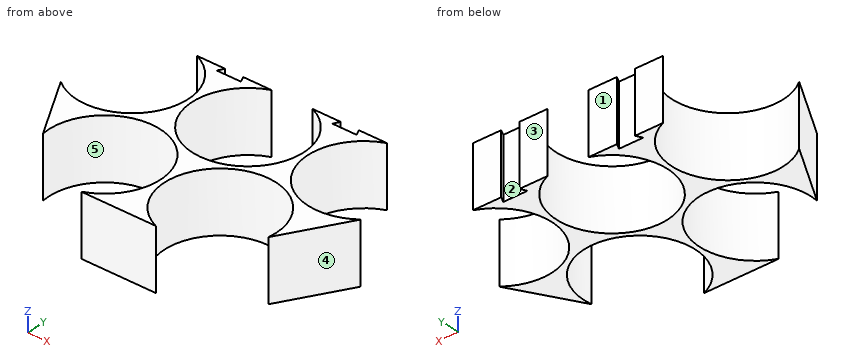
from build123d import *

# Parameters (mm, degrees)
BOSS_EXTRUDE1_DEPTH = 10
CUT_EXTRUDE1_DEPTH  = 11


with BuildPart() as part:
    # Sketch4 → Boss-Extrude1 (new body)
    with BuildSketch(Plane.XY):
        with BuildLine():
            Line((-47.308119418, -14.350263576), (-41.158711278, -25.001350911))
            ThreePointArc((-41.158711278, -25.001350911), (-27.519699416, -15.767887278), (-28.696607556, -32.196349849))
            Line((-28.696607556, -32.196349849), (-16.397791276, -32.196349849))
            ThreePointArc((-16.397791276, -32.196349849), (-17.574699416, -15.767887278), (-3.935687554, -25.001350911))
            Line((-3.935687554, -25.001350911), (2.213720586, -14.350263576))
            ThreePointArc((2.213720586, -14.350263576), (-11.375661988, -11.732764637), (-6.847791276, 1.344735363))
            Line((-6.847791276, 1.344735363), (-19.146607556, 1.344735363))
            ThreePointArc((-19.146607556, 1.344735363), (-22.547199416, -16.310264637), (-25.947791276, 1.344735363))
            Line((-25.947791276, 1.344735363), (-38.246607556, 1.344735363))
            ThreePointArc((-38.246607556, 1.344735363), (-33.718736844, -11.732764637), (-47.308119418, -14.350263576))
        make_face()
    extrude(amount=BOSS_EXTRUDE1_DEPTH)

    # Sketch5 → Cut-Extrude1 (cut, through all)
    with BuildSketch(Plane(origin=(0, 0, 0), x_dir=(-1, 0, 0), z_dir=(0, 0, -1))):
        Polygon((12.997199416, 1.344735363), (12.997199416, 0.344735363), (14.997199416, 0.344735363), (14.497199416, 1.344735363), align=None)
        Polygon((11.497199416, 1.344735363), (10.997199416, 0.344735363), (12.997199416, 0.344735363), (12.997199416, 1.344735363), align=None)
        Polygon((32.097199416, 0.344735363), (32.097199416, 1.344735363), (30.597199416, 1.344735363), (30.097199416, 0.344735363), align=None)
        Polygon((33.597199416, 1.344735363), (32.097199416, 1.344735363), (32.097199416, 0.344735363), (34.097199416, 0.344735363), align=None)
    extrude(amount=-CUT_EXTRUDE1_DEPTH, mode=Mode.SUBTRACT)


solid = part.part
Source: CAD feature listing. Evaluate the final solid. Frame: model axes, mm. Face numbers are marked on the shaded views. A direction names the side the tool comes from. Give positions to 0.01 mm unless a question says otherwise; leave off trailing zeros. Write each loop counter-clockwise with the first axis right and the second up, starting at its lowest first coordinate (ties: lowest second). Pieces come first, ordered by that corner, then holes. Notation, with made-up numbers: M 26.25,61.25 L 31.25,61.25 A26 cw 31.25,94.25 Z; hole C 63,-10.75 d8. An arc over 180 degrees is marked long. Return JSON: item names as keys, results as strings. Group by question number.
1) Material intervals for line 1 along X through (y, z) = (-19, 5.75); line 2 along X through (y, z) = (-20.5, 0.5); line 3 along X through (y, z) = (-8, 6), sorted ascending. Write a range as [from, to].
2) Cut plane C-C, the plane x = -8. Output: boundary loops of the cut face in (y, z).
3) Set-up query: the marked faces 1 and 2. Return all of +Z, -Z, +X, -X, +Y, -Y with unobstructed straight access to the full face (end or side cutting, diameter ignored); none if empty.
4) Cut plane B-B, the plane y = -17. Output: boundary loops of the cut face in (x, z), plus the area to 3 significant figures.
5) Cut plane A-A, the plane x = -27. Output: boundary loops of the cut face in (y, z), plus the area to 3 significant figures.
6) Cut plane D-D, the plane y = -3.5. Output: boundary loops of the cut face in (x, z).
7) Pull-direction query (X, two-part tool) for the marked faces 3, 4 and 5; classes: pulls with the +X half, pulls with the -X half, needs draft (parallel to the pull), parting line crosses it, or undercut.
8) Pin query (flat end, axial travel): P1, Ø11, axis at x = -3.45, y = -7.16, coming from the -Z side; P2, Ø1.5, axis at y = -27.5, z = 3, coming from the -X side (3 decimals); P3, Ø3, axis at x = -13.5, z = 2.5, coming from the +Y side; P4, Ø1.2, axis at x = -32, z = 4, coming from the +Y side. Return the tip coordinate at first contact, or that it passes through.
Recorded:
{
 "1": {"line 1": "x = [-44.62, -39.96], [-24.24, -20.86], [-5.14, -0.47]", "line 2": "x = [-43.76, -40.68], [-23.52, -21.58], [-4.42, -1.34]", "line 3": "x = [-32.53, -31.66], [-13.43, -12.56]"},
 "2": {"outline": "M -16.03,0 L -15.1,0 L -15.1,10 L -16.03,10 Z; M 0.79,0 L 1.34,0 L 1.34,10 L 0.79,10 Z"},
 "3": {"face 1": "+Z, -Z, +X, -X, +Y", "face 2": "+Z, -Z"},
 "4": {"outline": "M -45.78,0 L -38.34,0 L -38.34,10 L -45.78,10 Z; M -25.85,0 L -19.24,0 L -19.24,10 L -25.85,10 Z; M -6.75,0 L 0.68,0 L 0.68,10 L -6.75,10 Z", "area": "215 mm²"},
 "5": {"outline": "M -32.2,0 L -31.3,0 L -31.3,10 L -32.2,10 Z; M -16.09,0 L -15.15,0 L -15.15,10 L -16.09,10 Z; M 0.84,0 L 1.34,0 L 1.34,10 L 0.84,10 Z", "area": "23.3 mm²"},
 "6": {"outline": "M -33.25,0 L -30.94,0 L -30.94,10 L -33.25,10 Z; M -14.15,0 L -11.84,0 L -11.84,10 L -14.15,10 Z"},
 "7": {"face 3": "needs draft", "face 4": "pulls with the +X half", "face 5": "undercut"},
 "8": {"P1": "passes through", "P2": "stops at x = -24.155", "P3": "stops at y = 1.34", "P4": "stops at y = 0.34"}
}
